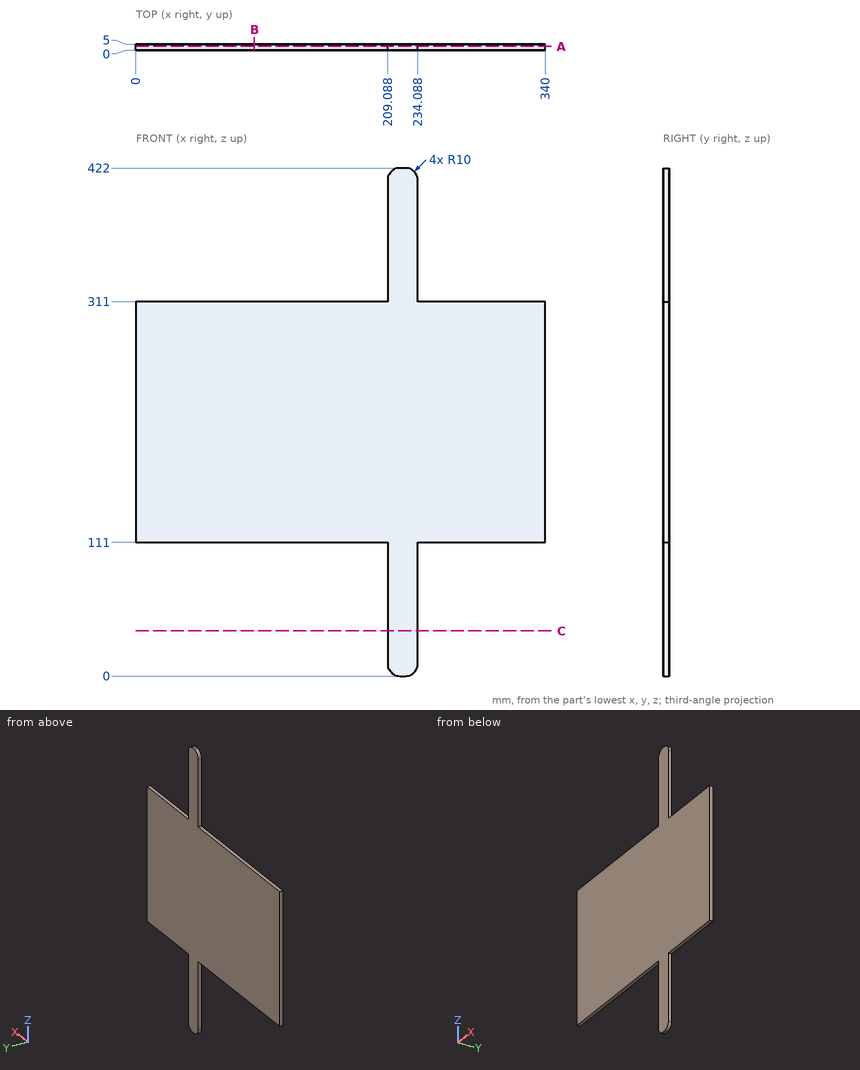
The drawing under review shows one solid part. Ordinate dimensions are in mm from its lowest x, y, z. Coordinates: 2 decimals unless noted, no trailing zeros. Loops run counter-clockwise (first coordinate to the right, second up) from the corner with the lowest first, then second, coordinate; pieces in that order, holes last. Notation, with made-up numbers: (23, 63.5) - (60, 63.5) arc R21 ccw to (60, 84.5) - close; hole circle Ø9 at (36.5, -37.75). An arc over 180 degrees is marked (long way). Return JSON: item names as keys, results as strings.
Item 1: Take a section at C-C (z = 37.5). Give the boundary of the cut face in (x, y), then the cut area to 3 significant figures.
Determined:
{"outline": "(209.09, 0) - (234.09, 0) - (234.09, 5) - (209.09, 5) - close", "area": "125 mm2"}
Item 2: Insertion check: pin 1 (1.5 mm diameter, centred on y = 1.5, z = 60.5, fed in from +X); pin 2 (5 mm diameter, centred on x = 229.5, z = 130.5, fed in from -Y); pin 3 (1.5 mm diameter, centred on y = 1.5, z = 375.5, fed in from -X); pin 4 (1 mm diameter, centred on x = 185.5, y = 2.5, fed in from -Z). Each pin has a flat end and moves straight along its axis. Give the tip position at first contact, or say it passes through.
Determined:
{"pin 1": "stops at x = 234.09", "pin 2": "stops at y = 0", "pin 3": "stops at x = 209.09", "pin 4": "stops at z = 111"}
Item 3: Take a section at A-A (y = 2.95). Give the boundary of the cut face in (x, z), then the cut area to 3 significant figures.
Determined:
{"outline": "(0, 111) - (209.09, 111) - (209.09, 10) arc R10 ccw to (219.09, 0) - (224.09, 0) arc R10 ccw to (234.09, 10) - (234.09, 111) - (340, 111) - (340, 311) - (234.09, 311) - (234.09, 412) arc R10 ccw to (224.09, 422) - (219.09, 422) arc R10 ccw to (209.09, 412) - (209.09, 311) - (0, 311) - close", "area": "73,500 mm2"}
Item 4: Take a section at B-B (x = 98.5). Give the boundary of the cut face in (y, z), then the cut area to 3 significant figures.
Determined:
{"outline": "(0, 111) - (5, 111) - (5, 311) - (0, 311) - close", "area": "1,000 mm2"}
Item 5: For line 1 (Z direction, x = 61.5, y = 0.85); line 2 (X direction, y = 2.35, z = 50), list the stretches that pass through material, from the lowest coordinate up.
Determined:
{"line 1": "z = 111 to 311", "line 2": "x = 209.09 to 234.09"}
